from build123d import *

# Parameters (mm, degrees)
SKETCH1_R           = 9.9
BOSS_EXTRUDE1_DEPTH = 2
SKETCH2_R           = 4.75
SKETCH2_R_2         = 2.75
BOSS_EXTRUDE2_DEPTH = 3.7
CUT_EXTRUDE1_REACH  = 17.117
SKETCH3_R           = 1.3
SKETCH3_R_2         = 1.45
CHAMFER1_SIZE       = 0.75
CHAMFER2_SIZE       = 0.2


with BuildPart() as part:
    # Sketch1 → Boss-Extrude1 (new body)
    with BuildSketch(Plane(origin=(0, 0, 0), x_dir=(1, 0, 0), z_dir=(0, 1, 0))):
        with Locations(Location((0, 0, 0), (0, 0, 270))):
            Circle(SKETCH1_R)
    extrude(amount=BOSS_EXTRUDE1_DEPTH)

    # Sketch2 → Boss-Extrude2 (add)
    with BuildSketch(Plane(origin=(0, 2, 0), x_dir=(1, 0, 0), z_dir=(0, 1, 0))):
        with Locations(Location((0, 0, 0), (0, 0, 270))):
            Circle(SKETCH2_R)
        with Locations(Location((0, 0, 0), (0, 0, 270))):
            Circle(SKETCH2_R_2, mode=Mode.SUBTRACT)
    extrude(amount=BOSS_EXTRUDE2_DEPTH)

    # Sketch3 → Cut-Extrude1 (cut, up to next)
    with BuildSketch(Plane.XZ, mode=Mode.PRIVATE) as cut_extrude1_sk1:
        with Locations(Location((-5, 5, 0), (0, 0, 270))):
            Circle(SKETCH3_R)
    cut_extrude1_tool1 = extrude(cut_extrude1_sk1.sketch, amount=-CUT_EXTRUDE1_REACH, mode=Mode.PRIVATE) & part.part
    # Sketch3 → Cut-Extrude1 (cut, up to next)
    with BuildSketch(Plane.XZ, mode=Mode.PRIVATE) as cut_extrude1_sk2:
        with Locations(Location((5, 5, 0), (0, 0, 270))):
            Circle(SKETCH3_R)
    cut_extrude1_tool2 = extrude(cut_extrude1_sk2.sketch, amount=-CUT_EXTRUDE1_REACH, mode=Mode.PRIVATE) & part.part
    # Sketch3 → Cut-Extrude1 (cut, up to next)
    with BuildSketch(Plane.XZ, mode=Mode.PRIVATE) as cut_extrude1_sk3:
        with Locations(Location((-5, -5, 0), (0, 0, 270))):
            Circle(SKETCH3_R)
    cut_extrude1_tool3 = extrude(cut_extrude1_sk3.sketch, amount=-CUT_EXTRUDE1_REACH, mode=Mode.PRIVATE) & part.part
    # Sketch3 → Cut-Extrude1 (cut, up to next)
    with BuildSketch(Plane.XZ, mode=Mode.PRIVATE) as cut_extrude1_sk4:
        with Locations(Location((5, -5, 0), (0, 0, 270))):
            Circle(SKETCH3_R)
    cut_extrude1_tool4 = extrude(cut_extrude1_sk4.sketch, amount=-CUT_EXTRUDE1_REACH, mode=Mode.PRIVATE) & part.part
    # Sketch3 → Cut-Extrude1 (cut, up to next)
    with BuildSketch(Plane.XZ, mode=Mode.PRIVATE) as cut_extrude1_sk5:
        with Locations(Location((0, 0, 0), (0, 0, 270))):
            Circle(SKETCH3_R_2)
    cut_extrude1_tool5 = extrude(cut_extrude1_sk5.sketch, amount=-CUT_EXTRUDE1_REACH, mode=Mode.PRIVATE) & part.part
    add(cut_extrude1_tool1.solids().sort_by_distance((-5, 0, 5))[0], mode=Mode.SUBTRACT)
    add(cut_extrude1_tool2.solids().sort_by_distance((5, 0, 5))[0], mode=Mode.SUBTRACT)
    add(cut_extrude1_tool3.solids().sort_by_distance((-5, 0, -5))[0], mode=Mode.SUBTRACT)
    add(cut_extrude1_tool4.solids().sort_by_distance((5, 0, -5))[0], mode=Mode.SUBTRACT)
    add(cut_extrude1_tool5.solids().sort_by_distance((0, 0, 0))[0], mode=Mode.SUBTRACT)

    # Chamfer1
    chamfer1_edges = [part.edges().sort_by_distance(p)[0] for p in [
        (0, 5.7, -2.75),
    ]]
    chamfer(chamfer1_edges, length=CHAMFER1_SIZE)

    # Chamfer2
    chamfer2_edges = [part.edges().sort_by_distance(p)[0] for p in [
        (0, 0, -9.9),
        (0, 2, -9.9),
    ]]
    chamfer(chamfer2_edges, length=CHAMFER2_SIZE)


solid = part.part
Geometry: final body of the model. Coordinates: model frame, mm. A direction names the side the tool comes from. Give positions to 0.01 mm unless a question says otherwise; leave off trailing zeros. Loops run counter-clockwise (first coordinate to the right, second up) from the corner with the lowest first, then second, coordinate; pieces in that order, holes last. Notation, with made-up numbers: M -33,-17.5 L -8,-17.5 A26 ccw -8,11.5 Z; hole C 21,56 d4. An arc over 180 degrees is marked long. Put each result on its own line as item: value.
1) First-contact query: P1, Ø3.5, axis at x = -5, z = -5, coming from the +Y side. Flat tip, straight axial feed; report the tip coordinate or a pass-through.
Computed values:
P1: stops at y = 2
2) Material intervals for L1, parallel to Z at x = 4.5, y = 0.6; L2, parallel to Y at x = 3, z = -7.75; L3, parallel to X at y = 0.7, z = -4.25, sorted ascending. Write a range as from..to.
Computed values:
L1: z = -8.82..-6.2, -3.8..3.8, 6.2..8.82
L2: y = 0..2
L3: x = -8.94..-6.06, -3.94..3.94, 6.06..8.94
3) Cut plane A-A, the plane x = 0. Return the cut outline in (y, z).
Computed values:
outline: M 0,-9.7 L 0.2,-9.9 L 1.8,-9.9 L 2,-9.7 L 2,-4.75 L 5.7,-4.75 L 5.7,-3.5 L 4.95,-2.75 L 2,-2.75 L 2,-1.45 L 0,-1.45 Z; M 0,1.45 L 2,1.45 L 2,2.75 L 4.95,2.75 L 5.7,3.5 L 5.7,4.75 L 2,4.75 L 2,9.7 L 1.8,9.9 L 0.2,9.9 L 0,9.7 Z
4) Cut plane D-D, the plane z = 6. Give the number of separate pieces and of enclosed holes in the cut face, plus the area to 3 significant figures.
Computed values:
separate pieces: 3
enclosed holes: 0
area: 24.8 mm^2
5) Mould query, pull axis X, two halves, no side actions, for faces 3 (the cylindrical face through (-2.685, 3.454, -0.596)), 4 (the cylindrical face through (2.974, 0.989, 9.443)), 5 (the flat face through (-2, 0, 0)). Classes: released by +X, released by -X, zero draft, split by the parting line, or undercut.
Computed values:
face 3: undercut
face 4: split by the parting line
face 5: zero draft
6) Cut plane C-C, the plane y = 3.8. Return the cut outline in (x, z), plus the area to 3 significant figures.
Computed values:
outline: C 0,0 d9.5; hole C 0,0 d5.5
area: 47.1 mm^2
7) Cut plane B-B, the plane z = 0. Return the cut outline in (x, y), plus the area to 3 significant figures.
Computed values:
outline: M -9.9,0.2 L -9.7,0 L -1.45,0 L -1.45,2 L -2.75,2 L -2.75,4.95 L -3.5,5.7 L -4.75,5.7 L -4.75,2 L -9.7,2 L -9.9,1.8 Z; M 1.45,0 L 9.7,0 L 9.9,0.2 L 9.9,1.8 L 9.7,2 L 4.75,2 L 4.75,5.7 L 3.5,5.7 L 2.75,4.95 L 2.75,2 L 1.45,2 Z
area: 48.0 mm^2
8) Reachability of faces 1 (the flat face through (2.3, 2, -4.4)), 2 (the cylindrical face through (-6.27, 0.99, -4.72)) from +Z, -Z, +X, -X, +Y, -Y: full face, straight path, thin tool, end or side. Return the list, or none.
Computed values:
face 1: +Y
face 2: +Y, -Y
